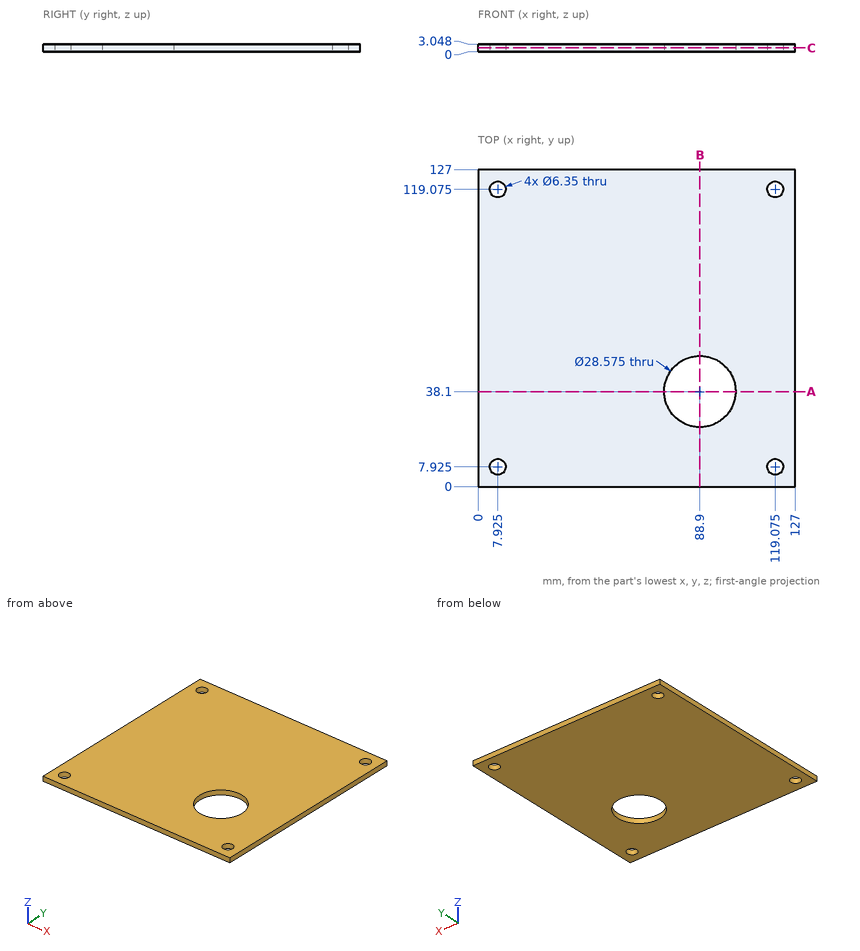
Print and shaded views of the part. All mm, measured from the part's lowest x, y and z. Give positions to 0.01 mm unless a question says otherwise; leave off trailing zeros. Loops run counter-clockwise (first coordinate to the right, second up) from the corner with the lowest first, then second, coordinate; pieces in that order, holes last. Notation, with made-up numbers: (-24.5, -23) -> (28.5, -23) arc R18 ccw to (28.5, -18) -> close; hole circle Ø7 at (20, -36). An arc over 180 degrees is marked (long way). Use a Markdown table: item, result.
1. Slice it at C-C (z = 1.45). Give the number of separate pieces and of enclosed holes in the cut face, plus the area to 3 significant figures.
Check result:
| item | result |
|---|---|
| separate pieces | 1 |
| enclosed holes | 5 |
| area | 15,400 mm^2 |
2. Slice it at B-B (x = 88.9). List the corners of the cut face in (y, z), plus the area to 3 significant figures.
Check result:
| item | result |
|---|---|
| outline | (0, 0) -> (23.81, 0) -> (23.81, 3.05) -> (0, 3.05) -> close; (52.39, 0) -> (127, 0) -> (127, 3.05) -> (52.39, 3.05) -> close |
| area | 300 mm^2 |
3. Wall check: L1, parallel to X at y = 119, z = 2.3; L2, parallel to X at y = 38.1, z = 1.55; L3, parallel to Y at x = 88.9, z = 0.75. Give the ranges that are in metal, low to high. Write a range as [from, to].
Check result:
| item | result |
|---|---|
| L1 | x = [0, 4.75], [11.1, 115.9], [122.25, 127] |
| L2 | x = [0, 74.61], [103.19, 127] |
| L3 | y = [0, 23.81], [52.39, 127] |
4. Slice it at A-A (y = 38.1). List the corners of the cut face in (x, z).
Check result:
| item | result |
|---|---|
| outline | (0, 0) -> (74.61, 0) -> (74.61, 3.05) -> (0, 3.05) -> close; (103.19, 0) -> (127, 0) -> (127, 3.05) -> (103.19, 3.05) -> close |
5. Flat gauge pin, fed straight in: pin 1 (4 mm diameter, centred on x = 7.92, y = 119.08, fed in from -Z). Where does the tip first touch, or does it go through?
Check result:
| item | result |
|---|---|
| pin 1 | passes through |
